Print and shaded views of the part. All mm, measured from the part's lowest x, y and z. Coordinates: 2 decimals unless noted, no trailing zeros. Loops run counter-clockwise (first coordinate to the right, second up) from the corner with the lowest first, then second, coordinate; pieces in that order, holes last. Notation, with made-up numbers: M 48,21.25 L 58,21.25 A15 cw 58,50.25 Z; hole C -34,71.5 d11. An arc over 180 degrees is marked long. Answer as a JSON object with one key per item and string values. Group by question number.
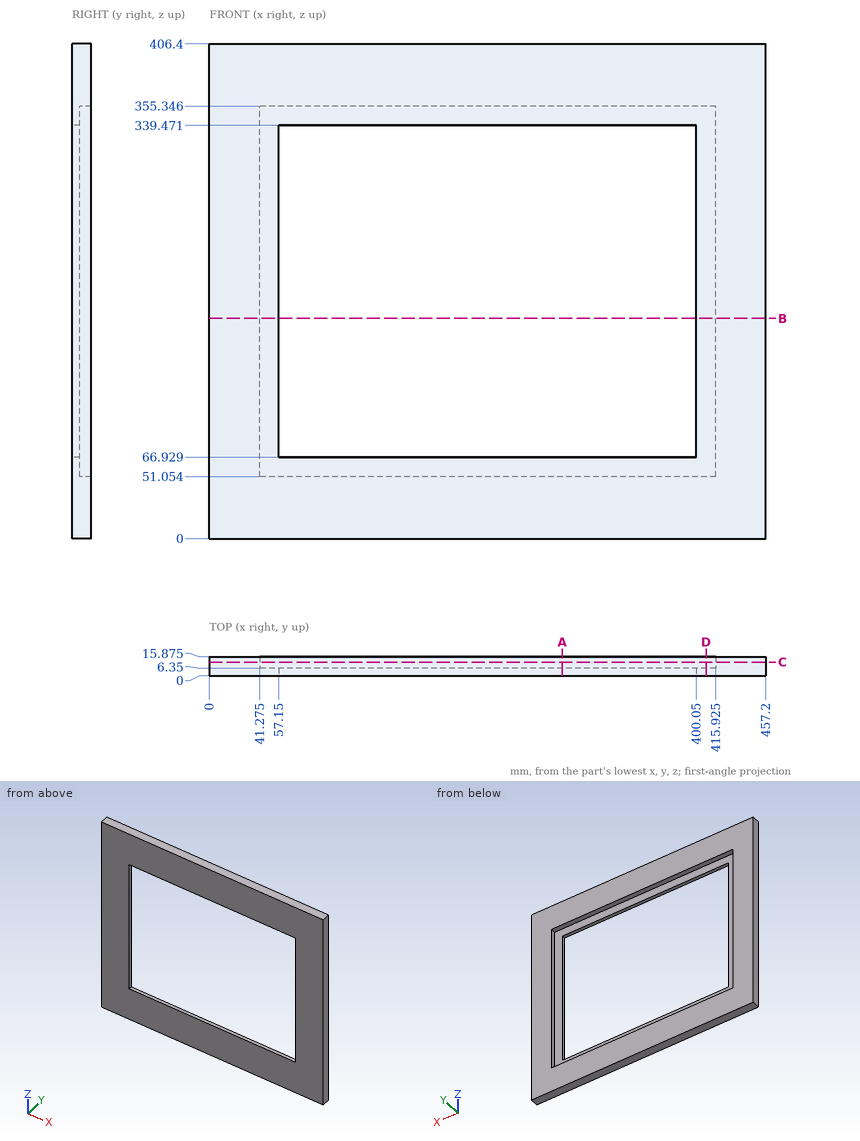
Item 1: Slice it at D-D, the plane x = 408. Write the cut outline in (y, z) (3 decimals), then the cut area to 3 significant figures.
Item 2: Slice it at B-B, the plane z = 181. Write the cut outline in (x, y) (3 decimals), then the cut area to 3 significant figures.
Item 3: Slice it at A-A, the plane x = 290. Write the cut outline in (y, z) (3 decimals).
Item 4: Drill centre lines: L1, parallel to Z at x = 93, y = 10; L2, parallel to X at y = 2, z = 211.5; L3, parallel to Z at x = 204, y = 5. Where is each one in solid material? Low to high. Write a range as from..to.
Item 5: Pin check, flat tip, straight feed: pin 1 (1 mm diameter, centred on y = 14, z = 334.5, fed in from -X). Stop position of the tip, or through.
Item 6: Slice it at C-C, the plane y = 11.5. Write the cut outline in (x, z) (3 decimals), then the cut area to 3 significant figures.
Computed:
{
 "1": {"outline": "M 0,0 L 15.875,0 L 15.875,51.054 L 6.35,51.054 L 6.35,355.346 L 15.875,355.346 L 15.875,406.4 L 0,406.4 Z", "area": "3,550 mm2"},
 "2": {"outline": "M 0,0 L 57.15,0 L 57.15,6.35 L 41.275,6.35 L 41.275,15.875 L 0,15.875 Z; M 400.05,0 L 457.2,0 L 457.2,15.875 L 415.925,15.875 L 415.925,6.35 L 400.05,6.35 Z", "area": "1,510 mm2"},
 "3": {"outline": "M 0,0 L 15.875,0 L 15.875,51.054 L 6.35,51.054 L 6.35,66.929 L 0,66.929 Z; M 0,339.471 L 6.35,339.471 L 6.35,355.346 L 15.875,355.346 L 15.875,406.4 L 0,406.4 Z"},
 "4": {"L1": "0..51.05, 355.35..406.4", "L2": "0..57.15, 400.05..457.2", "L3": "0..66.93, 339.47..406.4"},
 "5": {"pin 1": "x = 0"},
 "6": {"outline": "M 0,0 L 457.2,0 L 457.2,406.4 L 0,406.4 Z; hole M 41.275,51.054 L 415.925,51.054 L 415.925,355.346 L 41.275,355.346 Z", "area": "71,800 mm2"}
}
